```python
from build123d import *

# Parameters (mm, degrees)
BASE_DEPTH                    = 6
ESQUISSE10_R                  = 2.5
STEP_DEPTH                    = 223.656826754
ESQUISSE11_R                  = 15
ESQUISSE11_R_2                = 2.5
ENL_V_MAT_EXTRU_4_DEPTH       = 223.656826754
ESQUISSE12_R                  = 2.5
ENL_V_MAT_EXTRU_5_DEPTH       = 223.656826754
ESQUISSE14_R                  = 2.5
ENL_V_MAT_EXTRU_6_DEPTH       = 223.656826754
ESQUISSE15_R                  = 2.5
ENL_V_MAT_EXTRU_7_DEPTH       = 223.656826754
CONG_1_R                      = 10
SYM_TRIE4_DEPTH               = 6
ENL_V_MAT_EXTRU_13_DEPTH      = 223.656826754
ENL_V_MAT_EXTRU_13_DEPTH_BACK = 10
ESQUISSE16_R                  = 5


# Read off the part's stored shape, not the designer's step: Symétrie4
with BuildPart() as part:
    # Esquisse4 → Base (new body)
    with BuildSketch(Plane.XY):
        with BuildLine():
            Line((-176, 50), (-176, -50))
            Line((-176, -50), (-92.56776702, -136.25))
            Line((-92.56776702, -136.25), (92.56776702, -136.25))
            Line((92.56776702, -136.25), (176, -50))
            Line((176, -50), (176, 50))
            Line((176, 50), (96.5, 50))
            Line((96.5, 50), (96.5, 0))
            ThreePointArc((96.5, 0), (82.880465325, -32.880465325), (50, -46.5))
            Line((50, -46.5), (-50, -46.5))
            ThreePointArc((-50, -46.5), (-82.880465325, -32.880465325), (-96.5, 0))
            Line((-96.5, 0), (-96.5, 50))
            Line((-96.5, 50), (-176, 50))
        make_face()
    extrude(amount=BASE_DEPTH)

    # Esquisse10 → Step (cut, through all)
    with BuildSketch(Plane.XY):
        with Locations((-127, 26)):
            Circle(ESQUISSE10_R)
        with Locations((-153, 10)):
            Circle(ESQUISSE10_R)
        with Locations((-127, -6)):
            Circle(ESQUISSE10_R)
    step = extrude(amount=STEP_DEPTH, mode=Mode.SUBTRACT)

    # Step2: Step across plane
    add(step.mirror(Plane(origin=(0, 0, 0), x_dir=(0, 0, 1), z_dir=(1, 0, 0))), mode=Mode.SUBTRACT)

    # Esquisse11 → Enlèv. mat.-Extru.4 (cut, through all)
    with BuildSketch(Plane.XY):
        with Locations((0, -96.25)):
            Circle(ESQUISSE11_R)
        with Locations((-11.200595222, -76.85)):
            Circle(ESQUISSE11_R_2)
        with Locations((-11.200595222, -115.65)):
            Circle(ESQUISSE11_R_2)
        with Locations((22.401190445, -96.25)):
            Circle(ESQUISSE11_R_2)
    extrude(amount=ENL_V_MAT_EXTRU_4_DEPTH, mode=Mode.SUBTRACT)

    # Esquisse12 → Enlèv. mat.-Extru.5 (cut, through all)
    with BuildSketch(Plane.XY.offset(6)):
        with Locations((-77.25, -113.75)):
            Circle(ESQUISSE12_R)
        with Locations((-77.25, -82.75)):
            Circle(ESQUISSE12_R)
        with Locations((-57.25, -62.75)):
            Circle(ESQUISSE12_R)
        with Locations((-23.25, -62.75)):
            Circle(ESQUISSE12_R)
        with Locations((11.25, -115.75)):
            Circle(ESQUISSE12_R)
    extrude(amount=-ENL_V_MAT_EXTRU_5_DEPTH, mode=Mode.SUBTRACT)

    # Esquisse14 → Enlèv. mat.-Extru.6 (cut, through all)
    with BuildSketch(Plane.XY):
        with Locations((77.723139183, -94.064255673)):
            Circle(ESQUISSE14_R)
        with Locations((133.344627837, -36.564255673)):
            Circle(ESQUISSE14_R)
    extrude(amount=ENL_V_MAT_EXTRU_6_DEPTH, mode=Mode.SUBTRACT)

    # Esquisse15 → Enlèv. mat.-Extru.7 (cut, through all)
    with BuildSketch(Plane.XY.offset(6)):
        with Locations((-166, 40)):
            Circle(ESQUISSE15_R)
        with Locations((-126, 40)):
            Circle(ESQUISSE15_R)
        with Locations((126, 40)):
            Circle(ESQUISSE15_R)
        with Locations((166, 40)):
            Circle(ESQUISSE15_R)
    extrude(amount=-ENL_V_MAT_EXTRU_7_DEPTH, mode=Mode.SUBTRACT)

    # Congé1
    cong_1_edges = [part.edges().sort_by_distance(p)[0] for p in [
        (-96.5, 50, 3),
        (-92.56776702, -136.25, 3),
        (-176, -50, 3),
        (-176, 50, 3),
    ]]
    fillet(cong_1_edges, radius=CONG_1_R)

    # Symétrie4 outline → Symétrie4 (cut)
    with BuildSketch(Plane.XY):
        with BuildLine():
            Line((176, -50), (176, -45.954800825))
            ThreePointArc((176, -45.954800825), (175.270248109, -49.704800825), (173.1875, -52.907486907))
            Line((173.1875, -52.907486907), (176, -50))
        make_face()
        with BuildLine():
            ThreePointArc((96.5, 40), (99.428932188, 47.071067812), (106.5, 50))
            Line((106.5, 50), (96.5, 50))
            Line((96.5, 50), (96.5, 40))
        make_face()
        with BuildLine():
            ThreePointArc((166, 50), (173.071067812, 47.071067812), (176, 40))
            Line((176, 40), (176, 50))
            Line((176, 50), (166, 50))
        make_face()
        with BuildLine():
            Line((92.56776702, -136.25), (95.515525916, -133.202686082))
            ThreePointArc((95.515525916, -133.202686082), (92.231430788, -135.456705731), (88.328025916, -136.25))
            Line((88.328025916, -136.25), (92.56776702, -136.25))
        make_face()
    extrude(amount=SYM_TRIE4_DEPTH, mode=Mode.SUBTRACT)

    # Esquisse16 → Enlèv. mat.-Extru.13 (cut, two sides: drawn at the far end of the back side and taken through both)
    with BuildSketch(Plane.XY.offset(-ENL_V_MAT_EXTRU_13_DEPTH_BACK)):
        with Locations(Location((-85, -128.75, 0), (0, 0, 180))):
            Circle(ESQUISSE16_R)
        with Locations(Location((85, -128.75, 0), (0, 0, 180))):
            Circle(ESQUISSE16_R)
        with Locations(Location((-149.56929335, -62, 0), (0, 0, 180))):
            Circle(ESQUISSE16_R)
        with Locations(Location((149.56929335, -62, 0), (0, 0, 180))):
            Circle(ESQUISSE16_R)
    extrude(amount=ENL_V_MAT_EXTRU_13_DEPTH + ENL_V_MAT_EXTRU_13_DEPTH_BACK, mode=Mode.SUBTRACT)


solid = part.part
```
Input: part model. Units: mm. Frame: model coordinates. A direction names the side the tool comes from. Coordinates: 2 decimals unless noted, no trailing zeros. Loops run counter-clockwise (first coordinate to the right, second up) from the corner with the lowest first, then second, coordinate; pieces in that order, holes last. Notation, with made-up numbers: M 8,-14.5 L 48,-14.5 A26 ccw 48,19.5 Z; hole C 62,-5 d10. An arc over 180 degrees is marked long. Answer in a Markdown table with one row per item.
1. Draft query along X for faces 3 (the flat face through (-96.5, 20, 3)), 4 (the cylindrical face through (92.283, -135.435, 2.958)), 5 (the flat face through (-136, 50, 3)). Return one class per face: pulls with the +X half, pulls with the -X half, needs draft (parallel to the pull), parting line crosses it, or undercut.
Response:
| item | result |
|---|---|
| face 3 | undercut |
| face 4 | pulls with the +X half |
| face 5 | needs draft |
2. Material intervals for line 1 (Y direction, x = 0, z = 4.2); line 2 (X direction, y = -115, z = 2.2); line 3 (X direction, y = 36, z = 4.2), sorted ascending.
Response:
| item | result |
|---|---|
| line 1 | y = -136.25 to -111.25, -81.25 to -46.5 |
| line 2 | x = -113.12 to -79.42, -75.08 to -13.61, -8.79 to 8.87, 13.63 to 113.12 |
| line 3 | x = -176 to -96.5, 96.5 to 176 |
3. Section B-B, the plane z = 4. Count the separate pieces of the cut face and the enclosed holes in it, then the cut area to 3 significant figures.
Response:
| item | result |
|---|---|
| separate pieces | 1 |
| enclosed holes | 25 |
| area | 39,200 mm2 |
4. Reachability of faces 1 (the cylindrical face through (-144.574, -62.22, 2.958)), 2 (the flat face through (1, -46.5, 3)) from +Z, -Z, +X, -X, +Y, -Y: full face, straight path, thin tool, end or side. Return the list, or none.
Response:
| item | result |
|---|---|
| face 1 | +Z, -Z |
| face 2 | +Z, -Z, +Y |
5. Section A-A, the plane y = -29. Output: boundary loops of the cut face in (x, z), then the cut area to 3 significant figures.
Response:
| item | result |
|---|---|
| outline | M -176,0 L -86.35,0 L -86.35,6 L -176,6 Z; M 86.35,0 L 176,0 L 176,6 L 86.35,6 Z |
| area | 1,080 mm2 |
6. First-contact query: pin 1 (3 mm diameter, centred on x = -57.25, y = -62.75, fed in from +Z); pin 2 (3 mm diameter, centred on y = -91, z = 1, fed in from +X). Flat tips, straight axial feed; report the tip coordinate or a pass-through.
Response:
| item | result |
|---|---|
| pin 1 | passes through |
| pin 2 | stops at x = 137.79 |
